Source: three-view drawing plus pictorial views. Frame: mm from the lowest corner of the part. A direction names the side the tool comes from. Round coordinates to 2 decimals unless told otherwise and drop trailing zeros. Write each loop counter-clockwise with the first axis right and the second up, starting at its lowest first coordinate (ties: lowest second). Pieces come first, ordered by that corner, then holes. Notation, with made-up numbers: M 23.5,8 L 43.5,8 A9 cw 43.5,13 Z; hole C -9,33.5 d9. An arc over 180 degrees is marked long. Put each result on its own line as item: value. Start each with the question number.
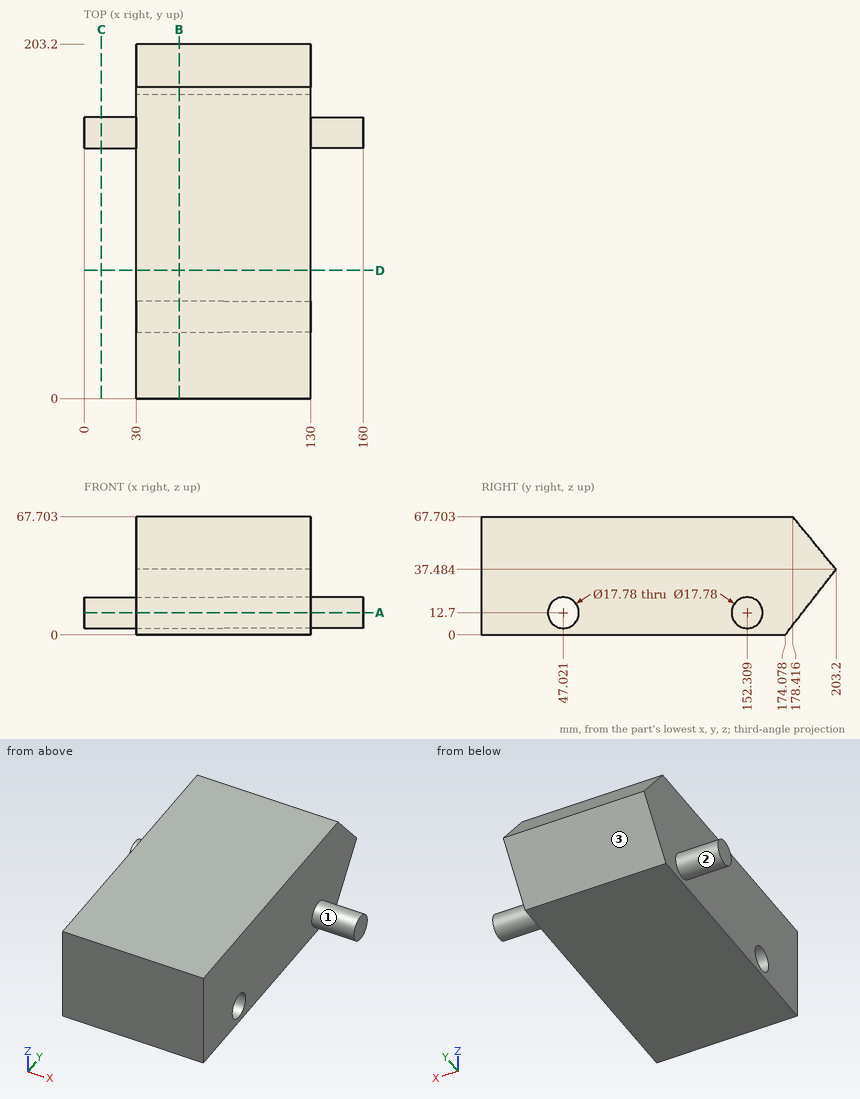
(1) Ray query, line 1 along X through (y, z) = (134.5, 57); line 2 along Y through (x, z) = (56.5, 16.5) (1 decimal); line 3 along Y through (x, z) = (97, 12) (1 decimal). Return the intervals inside material, ascending.
(2) Contact query for flat-ended pins moving along their axis: P1, Ø1.5, axis at y = 157, z = 23.5, coming from the +X side; P2, Ø1, axis at x = 85, y = 25, coming from the -Z side; P3, Ø10, axis at y = 29.5, z = 23, coming from the -X side. Output: stop coordinate, or through.
(3) Section query B-B (x = 54.5). Return loops of the section in (y, z), and give its area (3 significant figures).
(4) Section query A-A (z = 12.7). Return loops of the section in (x, y) (1 decimal).
(5) Section query D-D (y = 73.5). Return loops of the section in (x, z).
(6) Section query C-C (x = 10). Return loops of the section in (y, z).
(7) Access query for the marked faces 1, 2 and 3. Directions: +Z, -Z, +X, -X, +Y, -Y. A direction counts if a zero-diameter tool reaches every point of the face in a straight line with its end or side. Return the directions, or none.
Entries:
1. line 1: 30 to 130
1. line 2: 0 to 39, 55.1 to 186.9
1. line 3: 0 to 38.2, 55.9 to 183.4
2. P1: x = 130
2. P2: z = 0
2. P3: x = 30
3. outline: M 0,0 L 174.08,0 L 203.2,37.48 L 178.42,67.7 L 0,67.7 Z; hole C 47.02,12.7 d17.78
3. area: 12,600 mm2
4. outline: M 0,143.4 L 30,143.4 L 30,55.9 L 130,55.9 L 130,143.4 L 160,143.4 L 160,161.2 L 130,161.2 L 130,183.9 L 30,183.9 L 30,161.2 L 0,161.2 Z; M 30,0 L 130,0 L 130,38.1 L 30,38.1 Z
5. outline: M 30,0 L 130,0 L 130,67.7 L 30,67.7 Z
6. outline: C 152.31,12.7 d17.78
7. face 1: +X
7. face 2: -X
7. face 3: -Z, +X, -X, +Y
